from build123d import *

# Parameters (mm, degrees)
BOSS_EXTRUDE1_DEPTH = 16
SKETCH2_R           = 2.6
CUT_EXTRUDE1_DEPTH  = 4.8
SKETCH3_R           = 4.5
CUT_EXTRUDE2_DEPTH  = 10
CUT_EXTRUDE3_REACH  = 17
SKETCH4_R           = 1.6
SKETCH5_W           = 3
SKETCH5_H           = 3.5
CUT_EXTRUDE4_DEPTH  = 1.5
CHAMFER1_SIZE       = 1
SKETCH6_W           = 3.5
SKETCH6_H           = 9.5
CUT_EXTRUDE5_DEPTH  = 2
CHAMFER2_SIZE       = 1.5
FILLET1_R           = 1


with BuildPart() as part:
    # Sketch1 → Boss-Extrude1 (new body)
    with BuildSketch(Plane.XY):
        with BuildLine():
            Line((0, 0), (91.6, 0))
            Line((91.6, 0), (91.6, 4))
            Line((91.6, 4), (50, 4))
            ThreePointArc((50, 4), (42.928932188, 6.928932188), (40, 14))
            Line((40, 14), (34.5, 14))
            Line((34.5, 14), (33.5, 15))
            Line((33.5, 15), (26.5, 15))
            Line((26.5, 15), (25.5, 14))
            Line((25.5, 14), (14.5, 14))
            Line((14.5, 14), (13.5, 15))
            Line((13.5, 15), (6.5, 15))
            Line((6.5, 15), (5.5, 14))
            Line((5.5, 14), (0, 14))
            Line((0, 14), (0, 0))
        make_face()
    extrude(amount=-BOSS_EXTRUDE1_DEPTH)

    # Sketch2 → Cut-Extrude1 (cut)
    with BuildSketch(Plane(origin=(0, 15, 0), x_dir=(1, 0, 0), z_dir=(0, 1, 0))):
        with Locations((10, 8)):
            Circle(SKETCH2_R)
        with Locations((30, 8)):
            Circle(SKETCH2_R)
    extrude(amount=-CUT_EXTRUDE1_DEPTH, mode=Mode.SUBTRACT)

    # Sketch3 → Cut-Extrude2 (cut)
    with BuildSketch(Plane.XZ):
        with Locations((10, -8)):
            Circle(SKETCH3_R)
        with Locations((30, -8)):
            Circle(SKETCH3_R)
    extrude(amount=-CUT_EXTRUDE2_DEPTH, mode=Mode.SUBTRACT)

    # Sketch4 → Cut-Extrude3 (cut, up to next)
    with BuildSketch(Plane.XZ, mode=Mode.PRIVATE) as cut_extrude3_sk1:
        with Locations((88.6, -13)):
            Circle(SKETCH4_R)
    cut_extrude3_tool1 = extrude(cut_extrude3_sk1.sketch, amount=-CUT_EXTRUDE3_REACH, mode=Mode.PRIVATE) & part.part
    add(cut_extrude3_tool1.solids().sort_by_distance((88.6, 0, -13))[0], mode=Mode.SUBTRACT)
    # Sketch4 → Cut-Extrude3 (cut, up to next)
    with BuildSketch(Plane.XZ, mode=Mode.PRIVATE) as cut_extrude3_sk2:
        with Locations((69.6, -13)):
            Circle(SKETCH4_R)
    cut_extrude3_tool2 = extrude(cut_extrude3_sk2.sketch, amount=-CUT_EXTRUDE3_REACH, mode=Mode.PRIVATE) & part.part
    add(cut_extrude3_tool2.solids().sort_by_distance((69.6, 0, -13))[0], mode=Mode.SUBTRACT)

    # Sketch5 → Cut-Extrude4 (cut)
    with BuildSketch(Plane(origin=(0, 4, 0), x_dir=(1, 0, 0), z_dir=(0, 1, 0))):
        with Locations((74.1, 6.75)):
            Rectangle(SKETCH5_W, SKETCH5_H)
        with Locations((78.85, 6.75)):
            Rectangle(SKETCH5_W, SKETCH5_H)
        with Locations((83.6, 6.75)):
            Rectangle(SKETCH5_W, SKETCH5_H)
    extrude(amount=-CUT_EXTRUDE4_DEPTH, mode=Mode.SUBTRACT)

    # Chamfer1
    chamfer1_edges = [part.edges().sort_by_distance(p)[0] for p in [
        (72.6, 2.5, -6.75),
        (75.6, 2.5, -6.75),
        (77.35, 2.5, -6.75),
        (80.35, 2.5, -6.75),
        (82.1, 2.5, -6.75),
        (85.1, 2.5, -6.75),
    ]]
    chamfer(chamfer1_edges, length=CHAMFER1_SIZE)

    # Sketch6 → Cut-Extrude5 (cut)
    with BuildSketch(Plane(origin=(0, 4, 0), x_dir=(1, 0, 0), z_dir=(0, 1, 0))):
        with Locations((63.35, 7.75)):
            Rectangle(SKETCH6_W, SKETCH6_H)
    extrude(amount=-CUT_EXTRUDE5_DEPTH, mode=Mode.SUBTRACT)

    # Chamfer2
    chamfer2_edges = [part.edges().sort_by_distance(p)[0] for p in [
        (65.1, 2, -7.75),
        (61.6, 2, -7.75),
    ]]
    chamfer(chamfer2_edges, length=CHAMFER2_SIZE)

    # Fillet1
    fillet1_edges = [part.edges().sort_by_distance(p)[0] for p in [
        (91.6, 2, -16),
        (91.6, 2, 0),
        (0, 7, 0),
        (0, 7, -16),
    ]]
    fillet(fillet1_edges, radius=FILLET1_R)


solid = part.part
Read the model definition and answer for the solid it produces. Units are mm, in the model's axes. A direction names the side the tool comes from. Coordinates: 2 decimals unless noted, no trailing zeros. Loops run counter-clockwise (first coordinate to the right, second up) from the corner with the lowest first, then second, coordinate; pieces in that order, holes last.
Q1. The part is cut by section A-A on x = 69.6. Write down the section's boundary in (y, z), and give its area (3 significant figures).
Q2. The part is cut by section B-B on y = 8.75. Write down the section's boundary in (x, z), and give its area (3 significant figures).
Q3. Which of the six approach directions +Z, -Z, +X, -X, +Y, -Y give full straight-line access (tool end or side, diameter ignored) to faces 1 (the face through (14.16, 4.93, -9.72)), 2 (the face through (37, 14, -8)), 3 (the face through (3, 14, -8)), 4 (the face through (79, 3, -5))?
Q4. Consider probe 1 along X at (y, z) = (12.3, -8); probe 2 along X at (y, z) = (14.05, -8); probe 3 along Z at (x, y) = (10, 12.35). Determine where each line is inside the solid, lowest interval first.
Q5. The part is cut by section C-C on x = 10. Write down the section's boundary in (y, z), and give its area (3 significant figures).
Q6. Each of these flat-tipped pins is pushed along its axis until it touches: pin 1 Ø8 at (x, z) = (76, -10) entering from +Y; pin 2 Ø4.5 at (x, z) = (10, -8) entering from -Y; pin 3 Ø2 at (y, z) = (7.5, -13.5) entering from +X. Where does it stop, or does it pass through?
Q7. The mould has two halves that part along X. Classify faces 5 (the face through (91.6, 2, -8)), 6 (the face through (32, 15, -10)), 7 (the face through (74, 3, -5)): +X half, -X half, draft (parallel to the pull), parting line (faces both ways), or undercut.
Q8. The part is cut by section D-D on y = 13. Write down the section's boundary in (x, z), and give its area (3 significant figures).
Results below:
1. outline: (0, -16) - (4, -16) - (4, -14.6) - (0, -14.6) - close; (0, -11.4) - (4, -11.4) - (4, 0) - (0, 0) - close
1. area: 51.2 mm2
2. outline: (0, -15) arc R1 ccw to (1, -16) - (41.49, -16) - (41.49, 0) - (1, 0) arc R1 ccw to (0, -1) - close; hole circle Ø9 at (10, -8); hole circle Ø9 at (30, -8)
2. area: 536 mm2
3. face 1: -Y
3. face 2: +Z, -Z, +X, +Y
3. face 3: +Z, -Z, -X, +Y
3. face 4: +Y
4. probe 1: x = 0 to 7.4, 12.6 to 27.4, 32.6 to 40.15
4. probe 2: x = 5.55 to 7.4, 12.6 to 14.45, 25.55 to 27.4, 32.6 to 34.45
4. probe 3: z = -16 to -10.6, -5.4 to 0
5. outline: (0, -16) - (15, -16) - (15, -10.6) - (10.2, -10.6) - (10.2, -5.4) - (15, -5.4) - (15, 0) - (0, 0) - (0, -3.5) - (10, -3.5) - (10, -12.5) - (0, -12.5) - close
5. area: 125 mm2
6. pin 1: stops at y = 4
6. pin 2: stops at y = 10
6. pin 3: stops at x = 43.39
7. face 5: +X half
7. face 6: draft
7. face 7: undercut
8. outline: (0, -15) arc R1 ccw to (1, -16) - (40.05, -16) - (40.05, 0) - (1, 0) arc R1 ccw to (0, -1) - close; hole circle Ø5.2 at (10, -8); hole circle Ø5.2 at (30, -8)
8. area: 598 mm2
